Verification items for the finished model (mm, model axes). A direction names the side the tool comes from. Coordinates: 2 decimals unless noted, no trailing zeros. Order: outer loops, then holes, each group sorted by start corner. A loop starts at its lowest first (then second) coordinate and runs counter-clockwise, first axis right, second up. Notation, with made-up numbers: M 49.25,-20 L 108.25,-20 A19 cw 108.25,-2 Z; hole C 26.5,-16 d4. An arc over 180 degrees is marked long. Write item = value, one per line.
```python
from build123d import *

# Parameters (mm, degrees)
F1_DEPTH = 25.4


with BuildPart() as f1:
    # F0 (on Front) → F1 (new body)
    with BuildSketch(Plane.XZ):
        Polygon((-342.974587, 37.98175), (-342.974587, 12.58175), (-317.366544, 12.58175), (-317.366544, 37.964271), align=None)
        Polygon((-342.766544, 342.78175), (-342.974587, 37.98175), (-317.366544, 37.964271), (-317.366544, 177.68175), (-317.366544, 203.08175), (-317.366544, 342.78175), align=None)
        Polygon((1130.225413, 36.976212), (1155.625413, 36.958875), (1155.625413, 341.758875), (1130.225413, 341.758875), (1130.225413, 203.08175), (1130.225413, 177.68175), align=None)
        Polygon((-317.366544, 37.964271), (-317.366544, 12.58175), (1155.625413, 12.58175), (1155.625413, 36.958875), (1130.225413, 36.976212), (825.329516, 37.184319), (799.929528, 37.201656), (419.033727, 37.461638), (406.325413, 37.470312), (393.729435, 37.47891), (12.737937, 37.738957), (-12.566544, 37.756228), align=None)
        Polygon((-317.366544, 203.08175), (-317.366544, 177.68175), (-12.566544, 177.68175), (12.833456, 177.68175), (393.729435, 177.68175), (406.429435, 177.68175), (419.129435, 177.68175), (800.025413, 177.68175), (825.425413, 177.68175), (1130.225413, 177.68175), (1130.225413, 203.08175), align=None)
        Polygon((-12.566544, 177.68175), (-12.566544, 37.756228), (12.737937, 37.738957), (12.833456, 177.68175), align=None)
        Polygon((406.429435, 177.68175), (406.325413, 37.470312), (419.033727, 37.461638), (419.129435, 177.68175), align=None)
        Polygon((393.729435, 177.68175), (393.729435, 37.47891), (406.325413, 37.470312), (406.429435, 177.68175), align=None)
        Polygon((799.929528, 37.201656), (825.329516, 37.184319), (825.425413, 177.68175), (800.025413, 177.68175), align=None)
    extrude(amount=F1_DEPTH)


solid = f1.part
```
Item 1: Gauge pin test, flat ends, axial feed: pin 1 (12.5 mm diameter, centred on y = -7.5, z = 104.5, fed in from -X); pin 2 (5 mm diameter, centred on x = 374.5, y = -8, fed in from +Z); pin 3 (12.5 mm diameter, centred on x = 1144.5, y = -9.5, fed in from +Z). Record the tip position at first contact, or that the pin passes through.
Report:
pin_1 = -342.93
pin_2 = 203.08
pin_3 = 341.76
Item 2: Release check for a two-part mould opening along Z. For faces 1 (the flat face through (1143, -13, 341.759)), 2 (the flat face through (976, -13, 177.682)), 3 (the flat face through (1155.625, -13, 175)), 4 (the flat face through (-317.367, -13, 107)) record: pulls with the +Z half, pulls with the -Z half, needs draft (parallel to the pull), parting line crosses it, or undercut.
Report:
face_1 = pulls with the +Z half
face_2 = undercut
face_3 = needs draft
face_4 = undercut
Item 3: Sectioned sample at A-A, the plane y = -10.5. Enter the section's corners in (x, z), then the cut area to 3 significant figures.
Report:
outline = M -342.97,12.58 L 1155.63,12.58 L 1155.63,341.76 L 1130.23,341.76 L 1130.23,203.08 L -317.37,203.08 L -317.37,342.78 L -342.77,342.78 L -342.97,37.98 Z; hole M -317.37,37.96 L -12.57,37.76 L -12.57,177.68 L -317.37,177.68 Z; hole M 12.74,37.74 L 393.73,37.48 L 393.73,177.68 L 12.83,177.68 Z; hole M 419.03,37.46 L 799.93,37.2 L 800.03,177.68 L 419.13,177.68 Z; hole M 825.33,37.18 L 1130.23,36.98 L 1130.23,177.68 L 825.43,177.68 Z
area = 100,000 mm^2
Item 4: Scan lines: L1, parallel to X at y = -19.5, z = 82; L2, parallel to Z at x = 431.5, y = -6.5; L3, parallel to X at y = -16.5, z = 65.5. Record each from-to range of solid material in increasing order. Write a range as from..to.
Report:
L1 = -342.94..-317.37, -12.57..12.77, 393.73..419.06, 799.96..825.36, 1130.23..1155.63
L2 = 12.58..37.45, 177.68..203.08
L3 = -342.96..-317.37, -12.57..12.76, 393.73..419.05, 799.95..825.35, 1130.23..1155.63
Item 5: Sectioned sample at C-C, the plane z = 317. Enter the section's corners in (x, y).
Report:
outline = M -342.78,-25.4 L -317.37,-25.4 L -317.37,0 L -342.78,0 Z; M 1130.23,-25.4 L 1155.63,-25.4 L 1155.63,0 L 1130.23,0 Z
Item 6: Sectioned sample at B-B, the plane x = 336.5. Enter the section's corners in (y, z).
Report:
outline = M -25.4,12.58 L 0,12.58 L 0,37.52 L -25.4,37.52 Z; M -25.4,177.68 L 0,177.68 L 0,203.08 L -25.4,203.08 Z
Item 7: Tool access check on faces 5 (the flat face through (417, -13, 203.082)), 6 (the flat face through (201, -13, 177.682)), 7 (the flat face through (292, -25.4, 191)). Record the directions out of +Z, -Z, +X, -X, +Y, -Y that give a thin tool (end or side, any length) a straight path to the whole face; none if there is none.
Report:
face_5 = +Z, +Y, -Y
face_6 = +Y, -Y
face_7 = +Z, -Z, +X, -X, -Y
Item 8: Sectioned sample at D-D, the plane z = 84.5. Enter the section's corners in (x, y).
Report:
outline = M -342.94,-25.4 L -317.37,-25.4 L -317.37,0 L -342.94,0 Z; M -12.57,-25.4 L 12.77,-25.4 L 12.77,0 L -12.57,0 Z; M 393.73,-25.4 L 419.07,-25.4 L 419.07,0 L 393.73,0 Z; M 799.96,-25.4 L 825.36,-25.4 L 825.36,0 L 799.96,0 Z; M 1130.23,-25.4 L 1155.63,-25.4 L 1155.63,0 L 1130.23,0 Z
